Autodesk Inventor part; units mm, degrees
ref_plane "YZ Plane" through (0, 0, 0) normal (1, 0, 0) x (0, 1, 0)
ref_plane "XZ Plane" through (0, 0, 0) normal (0, 1, 0) x (-1, 0, 0)
ref_plane "XY Plane" through (0, 0, 0) normal (0, 0, 1) x (1, 0, 0)
sketch "Sketch1" plane through (0, 0, 0) normal (0, 0, 1) x (1, 0, 0)
  line L0 (0, 8.9862) -> (0, -66.0138)
  line L1 (0, 8.9862) -> (53, -66.0138)
  line L2 (0, -66.0138) -> (53, -66.0138)
  point P0 (0, 0)
  dimension "d0" = 75
  dimension "d39" = 53
sketch "Sketch2" plane through (0, 0, 0) normal (1, 0, 0) x (0, 1, 0)
  line L0 (4.5625, 0) -> (1.027, -3.5355)
  line L1 (1.9119, 0) -> (-2.0934, 0)
  point P0 (0, 0)
  dimension "d2" = 45
  dimension "d3" = 5
sweep "Sweep1" add profiles "Sketch1" path "Sketch2" path curves L0
sketch "Sketch3" plane through (0, -66.0138, 0) normal (-1, 0, 0) x (0, 0, 1)
  line L0 (0, 75) -> (0, 0)
  line L1 (0, 75) -> (-3.5355, 71.4645)
  line L2 (-3.5355, -3.5355) -> (-3.5355, 71.4645)
  line L3 (0, 0) -> (-3.5355, -3.5355)
  line L4 (0, 64.5) -> (-1.4142, 63.0858)
  line L5 (-1.4142, 63.0858) -> (-1.4142, 9.0858)
  line L6 (-1.4142, 9.0858) -> (0, 10.5)
  point P0 (0, 66.0138)
  dimension "d6" = 2
  dimension "d7" = 2
  dimension "d8" = 54
  dimension "d9" = 75
  dimension "d10" = 10.5
  dimension "d11" = 10.5
extrude "Extrusion1" add sketch "Sketch3" along normal blind 10 contours L0 L6 L5 L4
sketch "Sketch5" plane through (0, -56.9281, -1.4142) normal (0, 0, -1) x (-1, 0, 0)
  line L0 (0, 0) -> (0, 54)
  line L1 (0, 0) -> (10, 0)
  line L2 (10, 54) -> (10, 0)
  line L3 (0, 54) -> (10, 54)
  line L4 (4.25, 45.5) -> (6.25, 45.5)
  line L5 (6.25, 45.5) -> (6.25, 31.5)
  line L6 (6.25, 31.5) -> (4.25, 31.5)
  line L7 (4.25, 31.5) -> (4.25, 45.5)
  line L8 (4.25, 22.5) -> (6.25, 22.5)
  line L9 (6.25, 22.5) -> (6.25, 8.5)
  line L10 (6.25, 8.5) -> (4.25, 8.5)
  line L11 (4.25, 8.5) -> (4.25, 22.5)
  point P0 (0, 56.9281)
  dimension "d28" = 2
  dimension "d29" = 8.5
  dimension "d30" = 4.25
  dimension "d31" = 14
  dimension "d32" = 14
  dimension "d33" = 8.5
  dimension "d34" = 9
  dimension "d35" = 54
sketch "Sketch6" plane through (0, -69.5494, -3.5355) normal (-1, 0, 0) x (0, 0, 1)
  line L0 (3.5355, 14.0355) -> (2.1213, 12.6213)
  line L1 (2.1213, 12.6213) -> (2.1213, 66.6213)
  line L2 (2.1213, 66.6213) -> (3.5355, 68.0355)
  line L3 (3.5355, 78.5355) -> (3.5355, 68.0355)
  line L4 (3.5355, 78.5355) -> (0, 75)
  line L5 (0, 0) -> (0, 75)
  line L6 (3.5355, 3.5355) -> (0, 0)
  line L7 (3.5355, 14.0355) -> (3.5355, 3.5355)
  line L8 (3.5355, 68.0355) -> (2.1213, 66.6213)
  line L9 (2.1213, 66.6213) -> (2.1213, 12.6213)
  line L10 (2.1213, 12.6213) -> (3.5355, 14.0355)
  line L11 (3.5355, 14.0355) -> (3.5355, 68.0355)
  line L12 (2.1213, 64.596) -> (-1.4142, 61.0605)
  point P0 (3.5355, 69.5494)
  dimension "d36" = 5
sweep "Sweep2" add profiles "Sketch5" path "Sketch6" path curves L12 contours L4 L5 L6 L7 | L8 L9 L10 L11
equation "\"d10\" = -0.5 * d8 + 0.5 * d9"
equation "\"d32\" = d31"
equation "\"d33\" = d29"
properties part number "Rooft Extension Right Attachment"
Here's how the part is built. I have some questions about the finished solid (model axes, mm). A direction names the side the tool comes from. Round coordinates to 2 decimals unless told otherwise and drop trailing zeros. Loops run counter-clockwise (first coordinate to the right, second up) from the corner with the lowest first, then second, coordinate; pieces in that order, holes last.
1. If we section it at D-D on x = 24: Write out the boundary of the cut face in (y, z).
Answer list:
outline: (-69.55, -3.54) - (-28.51, -3.54) - (-24.98, 0) - (-66.01, 0) - close
2. If we section it at B-B on z = -2.5: Write out the boundary of the cut face in (x, y).
Answer list:
outline: (-6.25, -49.51) - (-4.25, -49.51) - (-4.25, -35.51) - (-6.25, -35.51) - close; (-6.25, -26.51) - (-4.25, -26.51) - (-4.25, -12.51) - (-6.25, -12.51) - close; (0, -68.51) - (53, -68.51) - (0, 6.49) - close
3. If I drill on line 1 along Z through (x, y) = (20, -48); line 2 along X through (y, z) = (-15, -2.8); line 3 along X through (y, z) = (-36.5, -2.5), over which ranges is the centre line in solid material (lowest first)?
Answer list:
line 1: z = -3.54 to 0
line 2: x = -6.25 to -4.25, 0 to 14.97
line 3: x = -6.25 to -4.25, 0 to 30.38
4. Which directions (+Z, -Z, +X, -X, +Y, -Y) give clear straight access to the entire face, cutting with the end or side of a thin tool? Please do faces 1 (the face through (14, -48, -3.536)), 2 (the face through (-6.25, -43, -3)), 3 (the face through (-5.264, -36.221, -3.207)).
Answer list:
face 1: -Z, +X, +Y, -Y
face 2: -Z, -X, +Y, -Y
face 3: -Z, -X
5. If we section it at C-C on y = -50: Write out the boundary of the cut face in (x, z).
Answer list:
outline: (-10, -1.41) - (0, -1.41) - (0, -3.54) - (39.19, -3.54) - (41.68, 0) - (-10, 0) - close; (-6.25, -4.95) - (-4.25, -4.95) - (-4.25, -2.99) - (-6.25, -2.99) - close
6. For P1, Ø10, axis at x = 26, y = -20, coming from the +Z side; P2, Ø1.8, axis at y = -45, z = -4, coming from the -X side; P3, Ø1, axis at y = -4, z = -2, coming from the -X side, each with a flat end and sliding along its axis, tell me the tip position at first contact or that it passes through.
Answer list:
P1: stops at z = 0
P2: stops at x = -6.25
P3: stops at x = 0
7. If we section it at A-A on y = -28: Write out the boundary of the cut face in (x, z).
Answer list:
outline: (-10, -1.41) - (0, -1.41) - (0, -3.54) - (23.64, -3.54) - (26.14, 0) - (-10, 0) - close; (-6.25, -4.95) - (-4.25, -4.95) - (-4.25, -3.99) - (-6.25, -3.99) - close
8. We'd pull the mould along Z, two halves only. Please class faces 4 (the face through (-6.25, -20, -3)), 5 (the face through (26.87, -30.83, -1.79)), 6 (the face through (-5.236, -27.221, -3.207)): +Z half, -Z half, draft (parallel to the pull), parting line (faces both ways), or undercut.
Answer list:
face 4: draft
face 5: -Z half
face 6: undercut
